Here's how the part is built. I have some questions about the finished solid (model axes, mm). A direction names the side the tool comes from. Coordinates: 2 decimals unless noted, no trailing zeros. Order: outer loops, then holes, each group sorted by start corner. A loop starts at its lowest first (then second) coordinate and runs counter-clockwise, first axis right, second up. Notation, with made-up numbers: (-9, -3.5) - (38, -3.5) arc R35 ccw to (38, 34.5) - close; hole circle Ø9 at (81, 21). An arc over 180 degrees is marked (long way). Use one line per item in the form item = value. Start each with the question number.
from build123d import *

# Parameters (mm, degrees)
SKETCH1_W                   = 45.8724
SKETCH1_H                   = 27.1272
BOSS_EXTRUDE1_DEPTH         = 22.1742
SKETCH2_R                   = 12.1539
BOSS_EXTRUDE2_DEPTH         = 13.5382
SKETCH3_R                   = 8.9662
BOSS_EXTRUDE3_DEPTH         = 1.2954
BOSS_EXTRUDE4_DEPTH         = 5.715
F_32_0_116_DIAMETER_HOLE1_D = 2.9464


with BuildPart() as part:
    # Sketch1 → Boss-Extrude1 (new body)
    with BuildSketch(Plane.XY):
        with Locations((22.9362, 13.5636)):
            Rectangle(SKETCH1_W, SKETCH1_H)
    extrude(amount=BOSS_EXTRUDE1_DEPTH)

    # Sketch2 → Boss-Extrude2 (add)
    with BuildSketch(Plane.XY.offset(22.1742)):
        with Locations((13.9065, 13.5636)):
            Circle(SKETCH2_R)
    extrude(amount=BOSS_EXTRUDE2_DEPTH)

    # Sketch3 → Boss-Extrude3 (add)
    with BuildSketch(Plane(origin=(0, 0, 0), x_dir=(-1, 0, 0), z_dir=(0, 0, -1))):
        with Locations((-11.2522, 13.5636)):
            Circle(SKETCH3_R)
    extrude(amount=BOSS_EXTRUDE3_DEPTH)

    # Sketch4 → Boss-Extrude4 (add)
    with BuildSketch(Plane(origin=(0, 0, -1.2954), x_dir=(-1, 0, 0), z_dir=(0, 0, -1))):
        with BuildLine():
            Line((-8.713438552, 15.8496), (-13.790961448, 15.8496))
            ThreePointArc((-13.790961448, 15.8496), (-14.6685, 13.5636), (-13.790961448, 11.2776))
            Line((-13.790961448, 11.2776), (-8.713438552, 11.2776))
            ThreePointArc((-8.713438552, 11.2776), (-8.06282103, 12.339276727), (-7.8359, 13.5636))
            ThreePointArc((-7.8359, 13.5636), (-8.06282103, 14.787923273), (-8.713438552, 15.8496))
        make_face()
    extrude(amount=BOSS_EXTRUDE4_DEPTH)

    # #32 (0.116) Diameter Hole1 (through all)
    with Locations(Plane(origin=(0, 0, 0), x_dir=(-1, 0, 0), z_dir=(0, 0, -1))):
        with Locations((-26.8224, 22.0472), (-26.8224, 5.08)):
            Hole(F_32_0_116_DIAMETER_HOLE1_D / 2)


solid = part.part
1) For pin 1 (8 mm diameter, centred on x = 7.5, y = 24, fed in from +Z); pin 2 (2.5 mm diameter, centred on x = 10.5, z = -4, fed in from -Y); pin 3 (4 mm diameter, centred on x = 26.82, y = 22.05, fed in from -Z); pin 4 (2.5 mm diameter, centred on x = 12, z = -3.5, fed in from +Y), each with a flat end and sliding along its axis, tell me the tip position at first contact or that it passes through.
2) Suppose I cut it at D-D, the plane y = 24.75. List the corners of the cut face in (x, z) for me, then the cut area to 3 significant figures.
3) Suppose I cut it at B-B, the plane y = 12.25. List the corners of the cut face in (x, z) for me.
4) Which directions (+Z, -Z, +X, -X, +Y, -Y) give clear straight access to the entire face, cutting with the end or side of a thin tool? Please do faces 4 (the flat face through (11, 15.85, -4)), 5 (the cylindrical face through (7.11, 5.61, -0.64)), 6 (the cylindrical face through (14.67, 13.6, -4.11)).
5) If we mould it in two halves opening along Y, with no side actions, what happens to faces 1 (the cylindrical face through (25.134, 8.909, 28.849)), 2 (the cylindrical face through (27.614, 6.322, 11.242)), 3 (the flat face through (23, 14, 0))? For each: pulls with the +Y half, pulls with the -Y half, needs draft (parallel to the pull), parting line crosses it, or undercut.
6) I need wall thicknesses on probe 1 along Z at (x, y) = (14.5, 9); probe 2 along Y at (x, z) = (14, 28); probe 3 along Z at (x, y) = (33, 13.5). Which ranges of each line are inside material? Lowest first, please. Write a range as [from, to].
7) Suppose I cut it at A-A, the plane x = 21. List the corners of the cut face in (y, z) for me, then the cut area to 3 significant figures.
8) Suppose I cut it at C-C, the plane z = 30. List the corners of the cut face in (x, y) for me.
From the geometry:
q1.pin_1 = 35.71
q1.pin_2 = 11.28
q1.pin_3 = 0
q1.pin_4 = 15.85
q2.outline = (0, 0) - (45.87, 0) - (45.87, 22.17) - (18.66, 22.17) - (18.66, 35.71) - (9.15, 35.71) - (9.15, 22.17) - (0, 22.17) - close
q2.area = 1,150 mm2
q3.outline = (0, 0) - (2.38, 0) - (2.38, -1.3) - (8.1, -1.3) - (8.1, -7.01) - (14.41, -7.01) - (14.41, -1.3) - (20.12, -1.3) - (20.12, 0) - (45.87, 0) - (45.87, 22.17) - (25.99, 22.17) - (25.99, 35.71) - (1.82, 35.71) - (1.82, 22.17) - (0, 22.17) - close
q4.face_4 = -Z, +X, -X, +Y
q4.face_5 = -Z
q4.face_6 = -Z, +X
q5.face_1 = parting line crosses it
q5.face_2 = undercut
q5.face_3 = needs draft
q6.probe_1 = [-1.3, 35.71]
q6.probe_2 = [1.41, 25.72]
q6.probe_3 = [0, 22.17]
q7.outline = (0, 0) - (27.13, 0) - (27.13, 22.17) - (23.43, 22.17) - (23.43, 35.71) - (3.69, 35.71) - (3.69, 22.17) - (0, 22.17) - close
q7.area = 869 mm2
q8.outline = circle Ø24.31 at (13.91, 13.56)
